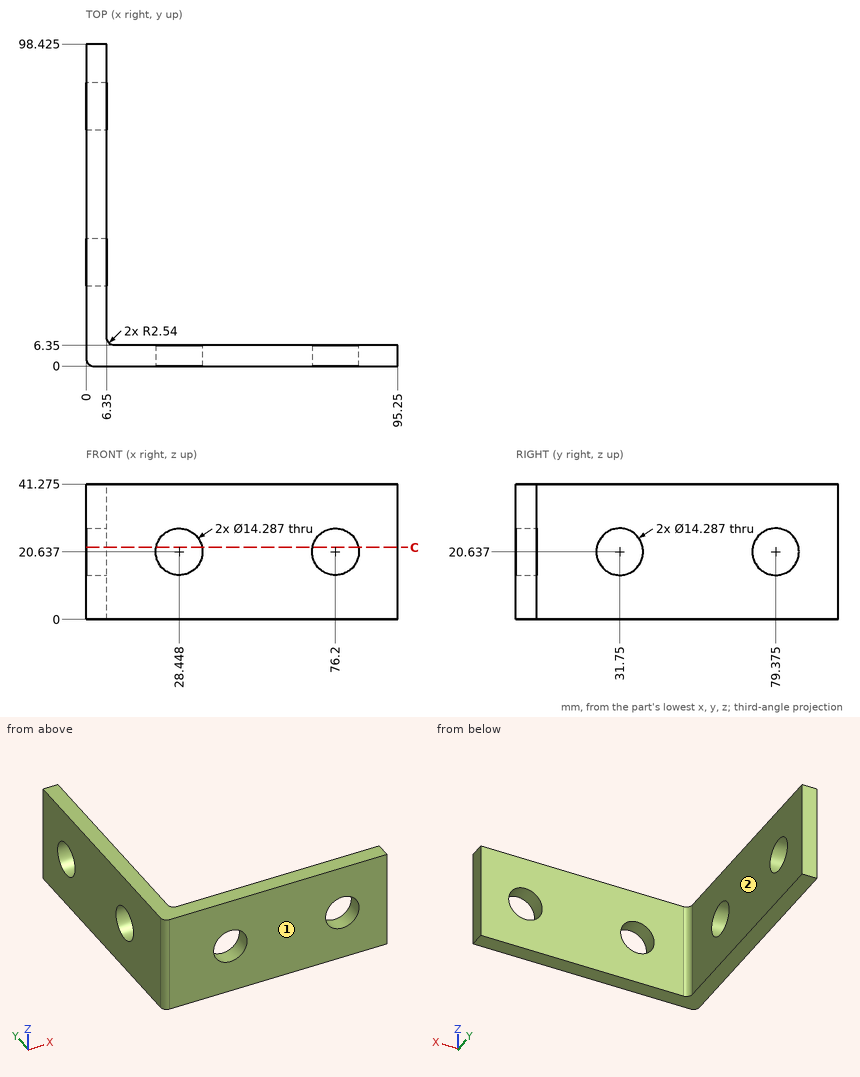
Geometry check sheet. Reference: drawing and pictorial views, mm from the part's lowest x, y, z. A direction names the side the tool comes from. Round coordinates to 2 decimals unless told otherwise and drop trailing zeros. Answer as a JSON object with one key per item and string values. Group by question number.
Item 1: Depth check by flat-ended pin: pin 1 Ø12.5 at (x, z) = (40.5, 13) entering from +Y; pin 2 Ø12 at (y, z) = (28.5, 11) entering from +X. Enter the tip coordinate at first touch or a pass-through.
Item 2: Thickness scan on line 1 along Z through (x, y) = (3.75, 31.75) (1 decimal); line 2 along Y through (x, z) = (21, 34); line 3 along Z through (x, y) = (3, 31) (1 decimal). Record the ranges inside material, lowest first.
Item 3: Cross-section at C-C, the plane z = 22. Count the separate pieces of the cut face and the enclosed holes in it.
Item 4: Set-up check for the marked faces 1 and 2: record each of +Z, -Z, +X, -X, +Y, -Y from which the full face is reachable in a straight line by a thin tool's end or side.
Determined:
{
 "1": {"pin 1": "stops at y = 6.35", "pin 2": "stops at x = 6.35"},
 "2": {"line 1": "z = 0 to 13.5, 27.8 to 41.3", "line 2": "y = 0 to 6.35", "line 3": "z = 0 to 13.5, 27.7 to 41.3"},
 "3": {"separate pieces": "5", "enclosed holes": "0"},
 "4": {"face 1": "+Z, -Z, +X, -X, -Y", "face 2": "+Z, -Z, +X, +Y"}
}
